Source: CAD feature listing. Evaluate the final solid. Frame: model axes, mm. Round coordinates to 2 decimals unless told otherwise and drop trailing zeros. Loops run counter-clockwise (first coordinate to the right, second up) from the corner with the lowest first, then second, coordinate; pieces in that order, holes last. Notation, with made-up numbers: M 79.5,80.25 L 116.5,80.25 A14 cw 116.5,101.25 Z; hole C 43,-8 d4. An arc over 180 degrees is marked long. Answer as CSV lines item,"result". Start each with the question number.
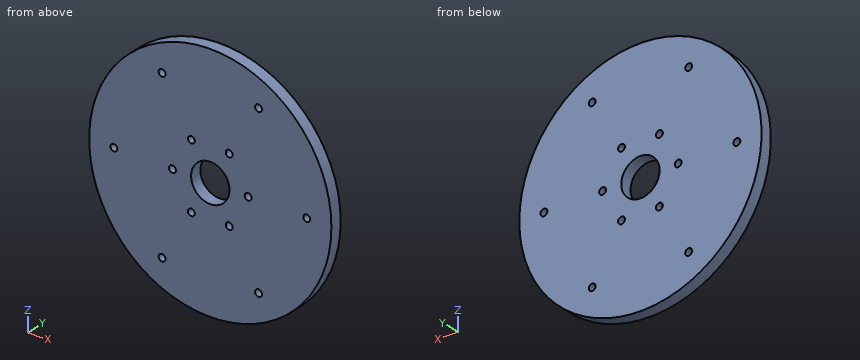
```python
from build123d import *

# Parameters (mm, degrees)
F0_R     = 76.2
F0_R_2   = 2.159
F0_R_3   = 12.065
F1_DEPTH = 7.62


with BuildPart() as f1:
    # F0 (on Front) → F1 (new body)
    with BuildSketch(Plane.XZ):
        Circle(F0_R)
        with Locations((-30.340516, -52.551315)):
            Circle(F0_R_2, mode=Mode.SUBTRACT)
        with Locations((-11.90625, -20.62223)):
            Circle(F0_R_2, mode=Mode.SUBTRACT)
        with Locations((30.340516, -52.551315)):
            Circle(F0_R_2, mode=Mode.SUBTRACT)
        with Locations((11.90625, -20.62223)):
            Circle(F0_R_2, mode=Mode.SUBTRACT)
        with Locations((-60.681032, 0)):
            Circle(F0_R_2, mode=Mode.SUBTRACT)
        with Locations((-23.8125, 0)):
            Circle(F0_R_2, mode=Mode.SUBTRACT)
        with Locations((-11.90625, 20.62223)):
            Circle(F0_R_2, mode=Mode.SUBTRACT)
        with Locations((-30.340516, 52.551315)):
            Circle(F0_R_2, mode=Mode.SUBTRACT)
        Circle(F0_R_3, mode=Mode.SUBTRACT)
        with Locations((23.8125, 0)):
            Circle(F0_R_2, mode=Mode.SUBTRACT)
        with Locations((11.90625, 20.62223)):
            Circle(F0_R_2, mode=Mode.SUBTRACT)
        with Locations((60.681032, 0)):
            Circle(F0_R_2, mode=Mode.SUBTRACT)
        with Locations((30.340516, 52.551315)):
            Circle(F0_R_2, mode=Mode.SUBTRACT)
    extrude(amount=-F1_DEPTH)


solid = f1.part
```
1) Section D-D, the plane z = 34.5. Return loops of the section in (x, y), and give its area (3 significant figures).
2) Section A-A, the plane x = 0. Return loops of the section in (y, z) (3 decimals), and give its area (3 significant figures).
3) Ray query, line 1 along Z through (x, y) = (0, 7.25) (3 decimals); line 2 along X through (y, z) = (3.25, 22); line 3 along X through (y, z) = (2.75, -53). Return the intervals inside material, ascending.
4) Section C-C, the plane y = 4.5. Give the number of separate pieces and of enclosed holes in the cut face, and give its area (3 significant figures).
5) Section B-B, the plane z = 0. Return loops of the section in (x, y) (1 decimal), and give its area (3 significant figures).
6) Contact query for flat-ended pins moving along their axis: pin 1 Ø3 at (x, y) = (-54.5, 1) entering from -Z; pin 2 Ø3 at (x, y) = (-37, 1.5) entering from +Z; pin 3 Ø4 at (x, y) = (53.5, 6) entering from +Z. Output: stop coordinate, or through.
Findings below:
1,outline,"M -67.94,0 L 67.94,0 L 67.94,7.62 L -67.94,7.62 Z"
1,area,"1,040 mm²"
2,outline,"M 0,-76.2 L 7.62,-76.2 L 7.62,-12.065 L 0,-12.065 Z; M 0,12.065 L 7.62,12.065 L 7.62,76.2 L 0,76.2 Z"
2,area,"977 mm²"
3,line 1,"-76.2 to -12.065, 12.065 to 76.2"
3,line 2,"-72.96 to -13.57, -10.24 to 10.24, 13.57 to 72.96"
3,line 3,"-54.75 to -32.45, -28.23 to 28.23, 32.45 to 54.75"
4,separate pieces,"1"
4,enclosed holes,"13"
4,area,"17,600 mm²"
5,outline,"M -76.2,0 L -62.8,0 L -62.8,7.6 L -76.2,7.6 Z; M -58.5,0 L -26,0 L -26,7.6 L -58.5,7.6 Z; M -21.7,0 L -12.1,0 L -12.1,7.6 L -21.7,7.6 Z; M 12.1,0 L 21.7,0 L 21.7,7.6 L 12.1,7.6 Z; M 26,0 L 58.5,0 L 58.5,7.6 L 26,7.6 Z; M 62.8,0 L 76.2,0 L 76.2,7.6 L 62.8,7.6 Z"
5,area,"846 mm²"
6,pin 1,"z = -54.75"
6,pin 2,"z = 67.43"
6,pin 3,"z = 56.16"
